from build123d import *

# Parameters (mm, degrees)
SKETCH1_W           = 228.6
SKETCH1_H           = 76.2
SKETCH1_R           = 4
SKETCH1_W_2         = 10
SKETCH1_H_2         = 30
BOSS_EXTRUDE1_DEPTH = 8
SKETCH1_3_W         = 10
SKETCH1_3_H         = 30
BOSS_EXTRUDE2_DEPTH = 40
FILLET1_R           = 3
SKETCH2_R           = 5
CUT_EXTRUDE1_DEPTH  = 211.575046005
FILLET2_R           = 15


with BuildPart() as part:
    # Sketch1 → Boss-Extrude1 (new body)
    # profile 1 of 5: a face of its own
    with BuildSketch(Plane.XY):
        Rectangle(SKETCH1_W, SKETCH1_H)
        with Locations((-101.6, -25.4)):
            Circle(SKETCH1_R, mode=Mode.SUBTRACT)
        with Locations((101.6, -25.4)):
            Circle(SKETCH1_R, mode=Mode.SUBTRACT)
        with Locations((101.6, 25.4)):
            Circle(SKETCH1_R, mode=Mode.SUBTRACT)
        with Locations((-101.6, 25.4)):
            Circle(SKETCH1_R, mode=Mode.SUBTRACT)
        with Locations((53.9, 0)):
            Rectangle(SKETCH1_W_2, SKETCH1_H_2, mode=Mode.SUBTRACT)
        with Locations((83.9, 0)):
            Rectangle(SKETCH1_W_2, SKETCH1_H_2, mode=Mode.SUBTRACT)
        with Locations((-83.9, 0)):
            Rectangle(SKETCH1_W_2, SKETCH1_H_2, mode=Mode.SUBTRACT)
        with Locations((-53.9, 0)):
            Rectangle(SKETCH1_W_2, SKETCH1_H_2, mode=Mode.SUBTRACT)
    # profile 2 of 5: a face of its own
    with BuildSketch(Plane.XY):
        with Locations((-53.9, 0)):
            Rectangle(SKETCH1_W_2, SKETCH1_H_2)
    # profile 3 of 5: a face of its own
    with BuildSketch(Plane.XY):
        with Locations((-83.9, 0)):
            Rectangle(SKETCH1_W_2, SKETCH1_H_2)
    # profile 4 of 5: a face of its own
    with BuildSketch(Plane.XY):
        with Locations((53.9, 0)):
            Rectangle(SKETCH1_W_2, SKETCH1_H_2)
    # profile 5 of 5: a face of its own
    with BuildSketch(Plane.XY):
        with Locations((83.9, 0)):
            Rectangle(SKETCH1_W_2, SKETCH1_H_2)
    extrude(amount=BOSS_EXTRUDE1_DEPTH)

    # Sketch1<3> → Boss-Extrude2 (add)
    with BuildSketch(Plane.XY):
        with Locations((-83.9, 0)):
            Rectangle(SKETCH1_3_W, SKETCH1_3_H)
        with Locations((-53.9, 0)):
            Rectangle(SKETCH1_3_W, SKETCH1_3_H)
        with Locations((83.9, 0)):
            Rectangle(SKETCH1_3_W, SKETCH1_3_H)
        with Locations((53.9, 0)):
            Rectangle(SKETCH1_3_W, SKETCH1_3_H)
    extrude(amount=-BOSS_EXTRUDE2_DEPTH)

    # Fillet1
    fillet1_edges = [part.edges().sort_by_distance(p)[0] for p in [
        (-83.9, 15, 0),
        (-88.9, 0, 0),
        (-83.9, -15, 0),
        (-48.9, 0, 0),
        (-53.9, 15, 0),
        (-53.9, -15, 0),
        (88.9, 0, 0),
        (83.9, -15, 0),
        (83.9, 15, 0),
        (53.9, -15, 0),
        (53.9, 15, 0),
        (48.9, 0, 0),
    ]]
    fillet(fillet1_edges, radius=FILLET1_R)

    # Sketch2 → Cut-Extrude1 (cut, through all)
    with BuildSketch(Plane.ZY.offset(88.9)):
        with Locations((-25, 0)):
            Circle(SKETCH2_R)
    extrude(amount=-CUT_EXTRUDE1_DEPTH, mode=Mode.SUBTRACT)

    # Fillet2
    fillet2_edges = [part.edges().sort_by_distance(p)[0] for p in [
        (53.9, 15, -40),
        (53.9, -15, -40),
        (83.9, 15, -40),
        (83.9, -15, -40),
        (-53.9, 15, -40),
        (-53.9, -15, -40),
        (-83.9, -15, -40),
        (-83.9, 15, -40),
    ]]
    fillet(fillet2_edges, radius=FILLET2_R - 0.0001)  # a hair under: the kernel refuses the full size


solid = part.part
Here's how the part is built. I have some questions about the finished solid (model axes, mm). A direction names the side the tool comes from. Round coordinates to 2 decimals unless told otherwise and drop trailing zeros. Order: outer loops, then holes, each group sorted by start corner. A loop starts at its lowest first (then second) coordinate and runs counter-clockwise, first axis right, second up. Notation, with made-up numbers: (84.25, 52.5) -> (119.25, 52.5) arc R28 cw to (119.25, 87.5) -> close; hole circle Ø10 at (89.5, 18). An arc over 180 degrees is marked (long way). Return JSON: item names as keys, results as strings.
Q1. If we section it at A-A on z = -18: List the corners of the cut face in (x, y) for me, plus the area to 3 significant figures.
Filled sheet:
{"outline": "(-88.9, -15) -> (-78.9, -15) -> (-78.9, 15) -> (-88.9, 15) -> close; (-58.9, -15) -> (-48.9, -15) -> (-48.9, 15) -> (-58.9, 15) -> close; (48.9, -15) -> (58.9, -15) -> (58.9, 15) -> (48.9, 15) -> close; (78.9, -15) -> (88.9, -15) -> (88.9, 15) -> (78.9, 15) -> close", "area": "1,200 mm^2"}
Q2. If we section it at D-D on x = 9: List the corners of the cut face in (y, z) for me.
Filled sheet:
{"outline": "(-38.1, 0) -> (38.1, 0) -> (38.1, 8) -> (-38.1, 8) -> close"}
Q3. Which directions (+Z, -Z, +X, -X, +Y, -Y) give clear straight access to the entire face, cutting with the end or side of a thin tool? Please do faces 4 (the flat face through (-88.9, 0, -17)), 5 (the flat face through (84, -15, -14)), 6 (the flat face through (-54, 15, -14)), 7 (the flat face through (48.9, 0, -17)).
Filled sheet:
{"face 4": "-Z, -X, +Y, -Y", "face 5": "-Z, +X, -X, -Y", "face 6": "-Z, +X, -X, +Y", "face 7": "-Z, +Y, -Y"}
Q4. If we section it at B-B on x = -101.6: List the corners of the cut face in (y, z) for me, plus the area to 3 significant figures.
Filled sheet:
{"outline": "(-38.1, 0) -> (-29.4, 0) -> (-29.4, 8) -> (-38.1, 8) -> close; (-21.4, 0) -> (21.4, 0) -> (21.4, 8) -> (-21.4, 8) -> close; (29.4, 0) -> (38.1, 0) -> (38.1, 8) -> (29.4, 8) -> close", "area": "482 mm^2"}
Q5. If we mould it in two halves opening along Z, with no side actions, what happens to faces 1 (the cylindrical face through (84, 0, -30)), 2 (the flat face through (-78.9, -0.3, -19.7)), 3 (the cylindrical face through (53.97, -10.72, -35.49))? For each: released by +Z, released by -Z, zero draft, split by the parting line, or undercut.
Filled sheet:
{"face 1": "undercut", "face 2": "zero draft", "face 3": "released by -Z"}
Q6. I need wall thicknesses on line 1 along X through (y, z) = (25, 1); line 2 along X through (y, z) = (-11.5, -5); line 3 along Y through (x, z) = (86, -25). Which ranges of each line are inside material? Lowest first, please. Write a range as from..to.
Filled sheet:
{"line 1": "x = -114.3..-105.58, -97.62..97.62, 105.58..114.3", "line 2": "x = -88.9..-78.9, -58.9..-48.9, 48.9..58.9, 78.9..88.9", "line 3": "y = -15..-5, 5..15"}
Q7. For pin 1 Ø6 at (x, z) = (89.5, -19) entering from +Y; pin 2 Ø8 at (x, z) = (86, -16) entering from -Y; pin 3 Ø1.5 at (y, z) = (10.5, -10) entering from +X, each with a flat end and sliding along its axis, tell me the tip position at first contact or that it passes through.
Filled sheet:
{"pin 1": "stops at y = 15", "pin 2": "stops at y = -15", "pin 3": "stops at x = 88.9"}
Q8. If we section it at C-C on y = 25.4: List the corners of the cut face in (x, z) for me.
Filled sheet:
{"outline": "(-114.3, 0) -> (-105.6, 0) -> (-105.6, 8) -> (-114.3, 8) -> close; (-97.6, 0) -> (97.6, 0) -> (97.6, 8) -> (-97.6, 8) -> close; (105.6, 0) -> (114.3, 0) -> (114.3, 8) -> (105.6, 8) -> close"}
